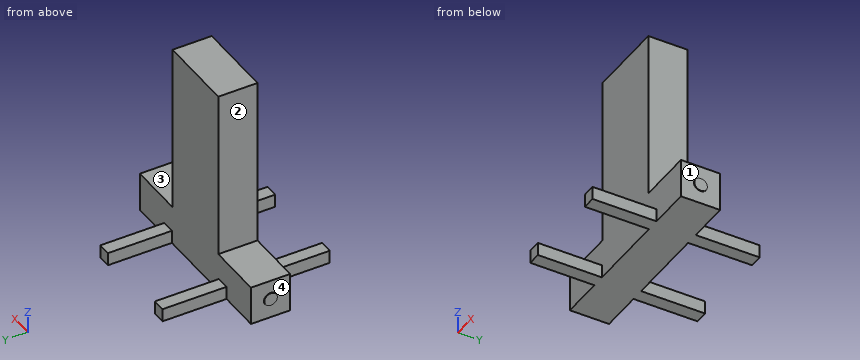
```python
from build123d import *

# Parameters (mm, degrees)
F0_W      = 19.05
F0_H      = 19.05
F1_DEPTH  = 46.228
F2_W      = 3.175
F2_H      = 6.35
F3_DEPTH  = 31.115
F4_W      = 3.175
F4_H      = 6.35
F5_DEPTH  = 31.115
F6_W      = 19.05
F6_H      = 19.05
F7_DEPTH  = 82.55
F8_R      = 3.175
F9_DEPTH  = 0.254
F10_R     = 3.175
F11_DEPTH = 0.254


with BuildPart() as f1:
    # F0 (on Right) → F1 (new body, symmetric)
    with BuildSketch(Plane.YZ):
        Rectangle(F0_W, F0_H)
    extrude(amount=F1_DEPTH, both=True)

    # F2 (on face) → F3 (join)
    with BuildSketch(Plane(origin=(0, 9.525, 0), x_dir=(-1, 0, 0), z_dir=(0, 1, 0))):
        with Locations((-21.1455, -6.35)):
            Rectangle(F2_W, F2_H)
        with Locations((-24.3205, -6.35)):
            Rectangle(F2_W, F2_H)
        with Locations((24.3205, -6.35)):
            Rectangle(F2_W, F2_H)
        with Locations((21.1455, -6.35)):
            Rectangle(F2_W, F2_H)
    extrude(amount=F3_DEPTH)

    # F4 (on face) → F5 (join)
    with BuildSketch(Plane.XZ.offset(9.525)):
        with Locations((-21.1455, -6.35)):
            Rectangle(F4_W, F4_H)
        with Locations((-24.3205, -6.35)):
            Rectangle(F4_W, F4_H)
        with Locations((24.3205, -6.35)):
            Rectangle(F4_W, F4_H)
        with Locations((21.1455, -6.35)):
            Rectangle(F4_W, F4_H)
    extrude(amount=F5_DEPTH)

    # F6 (on face) → F7 (join)
    with BuildSketch(Plane.XY.offset(9.525)):
        with Locations((9.525, 0)):
            Rectangle(F6_W, F6_H)
        with Locations((-9.525, 0)):
            Rectangle(F6_W, F6_H)
    extrude(amount=F7_DEPTH)

    # F8 (on face) → F9 (join)
    with BuildSketch(Plane(origin=(-46.228, 0, 0), x_dir=(0, -1, 0), z_dir=(-1, 0, 0))):
        Circle(F8_R)
    extrude(amount=F9_DEPTH)

    # F10 (on face) → F11 (join)
    with BuildSketch(Plane.YZ.offset(46.228)):
        Circle(F10_R)
    extrude(amount=F11_DEPTH)


solid = f1.part
```
Verification items for the finished model (mm, model axes). Face numbers are marked on the shaded views. A direction names the side the tool comes from. Round coordinates to 2 decimals unless told otherwise and drop trailing zeros. Order: outer loops, then holes, each group sorted by start corner. A loop starts at its lowest first (then second) coordinate and runs counter-clockwise, first axis right, second up. Notation, with made-up numbers: (-3.75, 26) -> (27.25, 26) arc R26 ccw to (27.25, 58) -> close; hole circle Ø1 at (35, 69). An arc over 180 degrees is marked (long way). Put each result on its own line as item: value. Start each with the question number.
(1) Section check C-C (y = 7). Enter the section's corners in (x, z) (3 decimals).
(2) Tool access check on the marked faces 1, 2, 3 and 4. Record the directions out of +Z, -Z, +X, -X, +Y, -Y that give a thin tool (end or side, any length) a straight path to the whole face; none if there is none.
(3) Section check B-B (z = 0). Enter the section's corners in (x, y) (3 decimals), then the cut area to 3 significant figures.
(4) Depth check by flat-ended pin: pin 1 Ø7 at (y, z) = (28.5, -7) entering from +X; pin 2 Ø1.9 at (x, y) = (-24, -27) entering from +Z (3 decimals); pin 3 Ø5 at (y, z) = (-27, -5.5) entering from -X. Enter the tip coordinate at first touch or a pass-through.
(5) Section check D-D (x = 41). Enter the section's corners in (y, z) (3 decimals), then the cut area to 3 significant figures.
(6) Material ranges on line 1 along Z through (x, y) = (25.5, 33.5) (3 decimals); line 2 along X through (y, z) = (-8, -3); line 3 along Z through (x, y) = (-33.5, 7) (3 decimals), recorded low to high.
(7) Section check A-A (y = 19). Enter the section's corners in (x, z) (3 decimals).
Completed:
1. outline: (-46.228, -9.525) -> (46.228, -9.525) -> (46.228, 9.525) -> (19.05, 9.525) -> (19.05, 92.075) -> (-19.05, 92.075) -> (-19.05, 9.525) -> (-46.228, 9.525) -> close
2. face 1: +X
2. face 2: +Z, -X, +Y, -Y
2. face 3: +Z, +X, +Y, -Y
2. face 4: -X
3. outline: (-46.482, -3.175) -> (-46.228, -3.175) -> (-46.228, -9.525) -> (46.228, -9.525) -> (46.228, -3.175) -> (46.482, -3.175) -> (46.482, 3.175) -> (46.228, 3.175) -> (46.228, 9.525) -> (-46.228, 9.525) -> (-46.228, 3.175) -> (-46.482, 3.175) -> close
3. area: 1,760 mm2
4. pin 1: stops at x = 25.91
4. pin 2: stops at z = -3.175
4. pin 3: stops at x = -25.91
5. outline: (-9.525, -9.525) -> (9.525, -9.525) -> (9.525, 9.525) -> (-9.525, 9.525) -> close
5. area: 363 mm2
6. line 1: z = -9.525 to -3.175
6. line 2: x = -46.23 to 46.23
6. line 3: z = -9.525 to 9.525
7. outline: (-25.908, -9.525) -> (-19.558, -9.525) -> (-19.558, -3.175) -> (-25.908, -3.175) -> close; (19.558, -9.525) -> (25.908, -9.525) -> (25.908, -3.175) -> (19.558, -3.175) -> close
